```python
from build123d import *

# Parameters (mm, degrees)
SKETCH1_W           = 25.4
SKETCH1_H           = 19.05
BOSS_EXTRUDE1_DEPTH = 101.6
SKETCH2_R           = 6.35
CUT_EXTRUDE1_DEPTH  = 101.6
SKETCH3_W           = 25.4
SKETCH3_H           = 12.7
BOSS_EXTRUDE2_DEPTH = 19.05
SKETCH5_W           = 6.35
SKETCH5_H           = 19.05
BOSS_EXTRUDE4_DEPTH = 9.525
SKETCH8_W           = 25.4
SKETCH8_H           = 12.7
BOSS_EXTRUDE5_DEPTH = 19.05
SKETCH9_W           = 6.35
SKETCH9_H           = 19.05
BOSS_EXTRUDE6_DEPTH = 9.525


with BuildPart() as part:
    # Sketch1 → Boss-Extrude1 (new body)
    with BuildSketch(Plane.XY):
        with Locations((-12.7, 9.525)):
            Rectangle(SKETCH1_W, SKETCH1_H)
    extrude(amount=BOSS_EXTRUDE1_DEPTH)

    # Sketch2 → Cut-Extrude1 (cut)
    with BuildSketch(Plane.XY.offset(101.6)):
        with Locations((-12.7, 9.525)):
            Circle(SKETCH2_R)
    extrude(amount=-CUT_EXTRUDE1_DEPTH, mode=Mode.SUBTRACT)

    # Sketch3 → Boss-Extrude2 (add)
    with BuildSketch(Plane(origin=(0, 19.05, 0), x_dir=(1, 0, 0), z_dir=(0, 1, 0))):
        with Locations((-38.1, -95.25)):
            Rectangle(SKETCH3_W, SKETCH3_H)
    extrude(amount=-BOSS_EXTRUDE2_DEPTH)

    # Sketch5 → Boss-Extrude4 (add)
    with BuildSketch(Plane.XY.offset(101.6)):
        with Locations((-47.625, 9.525)):
            Rectangle(SKETCH5_W, SKETCH5_H)
    extrude(amount=BOSS_EXTRUDE4_DEPTH)

    # Sketch8 → Boss-Extrude5 (add)
    with BuildSketch(Plane(origin=(0, 19.05, 0), x_dir=(1, 0, 0), z_dir=(0, 1, 0))):
        with Locations((12.7, -6.35)):
            Rectangle(SKETCH8_W, SKETCH8_H)
    extrude(amount=-BOSS_EXTRUDE5_DEPTH)

    # Sketch9 → Boss-Extrude6 (add)
    with BuildSketch(Plane(origin=(0, 0, 0), x_dir=(-1, 0, 0), z_dir=(0, 0, -1))):
        with Locations((-22.225, 9.525)):
            Rectangle(SKETCH9_W, SKETCH9_H)
    extrude(amount=BOSS_EXTRUDE6_DEPTH)


solid = part.part
```
Source: CAD feature listing. Evaluate the final solid. Frame: model axes, mm. A direction names the side the tool comes from. Round coordinates to 2 decimals unless told otherwise and drop trailing zeros. Loops run counter-clockwise (first coordinate to the right, second up) from the corner with the lowest first, then second, coordinate; pieces in that order, holes last.
1. Ray query, L1, parallel to Y at x = -12.7, z = 44 (3 decimals); L2, parallel to X at y = 9.5, z = 68.5; L3, parallel to Z at x = 13, y = 16. Return the intervals inside material, ascending.
2. Section query C-C on z = 58. Output: boundary loops of the cut face in (x, y) (3 decimals), and give its area (3 significant figures).
3. Section query B-B on y = 13. Output: boundary loops of the cut face in (x, z) (3 decimals).
4. Contact query for flat-ended pins moving along their axis: pin 1 (4 mm diameter, centred on y = 12.5, z = 38, fed in from -X); pin 2 (5 mm diameter, centred on x = 8, y = 10, fed in from +Z); pin 3 (8 mm diameter, centred on y = 13, z = 36, fed in from +X). Output: stop coordinate, or through.
5. Section query D-D on x = -33.5. Output: boundary loops of the cut face in (y, z), and give its area (3 significant figures).
6. Section query A-A on x = -12.7. Output: boundary loops of the cut face in (y, z) (3 decimals).
7. Mould query, pull axis Y, two halves, no side actions, for faces 4 (the flat face through (-10, 19.05, 51)), 5 (the flat face through (-10, 0, 51)), 6 (the cylindrical face through (-9.77, 3.89, 51.51)), 7 (the flat face through (0, 9, 57)). Classes: released by +Y, released by -Y, zero draft, split by the parting line, or undercut.
8. Access query for faces 1 (the flat face through (-25.4, 9, 44)), 2 (the flat face through (-23, 10, 101.6)), 3 (the flat face through (22, 10, -9.525)). Directions: +Z, -Z, +X, -X, +Y, -Y. A direction counts if a zero-diameter tool reaches every point of the face in a straight line with its end or side. Return the directions, or none.
Answers below:
1. L1: y = 0 to 3.175, 15.875 to 19.05
1. L2: x = -25.4 to -19.05, -6.35 to 0
1. L3: z = 0 to 12.7
2. outline: (-25.4, 0) - (0, 0) - (0, 19.05) - (-25.4, 19.05) - close; hole circle Ø12.7 at (-12.7, 9.525)
2. area: 357 mm2
3. outline: (-50.8, 88.9) - (-25.4, 88.9) - (-25.4, 0) - (-18.015, 0) - (-18.015, 101.6) - (-44.45, 101.6) - (-44.45, 111.125) - (-50.8, 111.125) - close; (-7.385, 0) - (19.05, 0) - (19.05, -9.525) - (25.4, -9.525) - (25.4, 12.7) - (0, 12.7) - (0, 101.6) - (-7.385, 101.6) - close
4. pin 1: stops at x = -25.4
4. pin 2: stops at z = 12.7
4. pin 3: stops at x = 0
5. outline: (0, 88.9) - (19.05, 88.9) - (19.05, 101.6) - (0, 101.6) - close
5. area: 242 mm2
6. outline: (0, 0) - (3.175, 0) - (3.175, 101.6) - (0, 101.6) - close; (15.875, 0) - (19.05, 0) - (19.05, 101.6) - (15.875, 101.6) - close
7. face 4: released by +Y
7. face 5: released by -Y
7. face 6: undercut
7. face 7: zero draft
8. face 1: -Z, -X, +Y, -Y
8. face 2: +Z, +X, +Y, -Y
8. face 3: -Z, +X, -X, +Y, -Y
